from build123d import *

# Parameters (mm, degrees)
BOSS_EXTRUDE1_DEPTH  = 15
CUT_EXTRUDE1_START   = -4
SKETCH2_R            = 3
CUT_EXTRUDE1_DEPTH   = 17
M3_CLEARANCE_HOLE1_D = 3.4
FILLET2_R            = 2


with BuildPart() as part:
    # Sketch1 → Boss-Extrude1 (new body, symmetric)
    with BuildSketch(Plane(origin=(0, 0, 0), x_dir=(1, 0, 0), z_dir=(0, 1, 0))):
        Polygon((0, 0), (0, -7.5), (-20, 12.5), (-20, 25), (0, 5), align=None)
    extrude(amount=BOSS_EXTRUDE1_DEPTH, both=True)

    # Sketch2 → Cut-Extrude1 (cut, through all)
    with BuildSketch(Plane(origin=(0, 0, 0), x_dir=(0, 0, -1), z_dir=(1, 0, 0)).offset(CUT_EXTRUDE1_START)):
        with Locations((0, 10)):
            Circle(SKETCH2_R)
        with Locations((0, -10)):
            Circle(SKETCH2_R)
    extrude(amount=-CUT_EXTRUDE1_DEPTH, mode=Mode.SUBTRACT)

    # M3 Clearance Hole1 (through all)
    with Locations(Plane.ZY.offset(4)):
        with Locations((0, 10), (0, -10)):
            Hole(M3_CLEARANCE_HOLE1_D / 2)

    # Fillet2
    fillet2_edges = [part.edges().sort_by_distance(p)[0] for p in [
        (-20, 0, -12.5),
        (-20, 0, -25),
    ]]
    fillet(fillet2_edges, radius=FILLET2_R)


solid = part.part
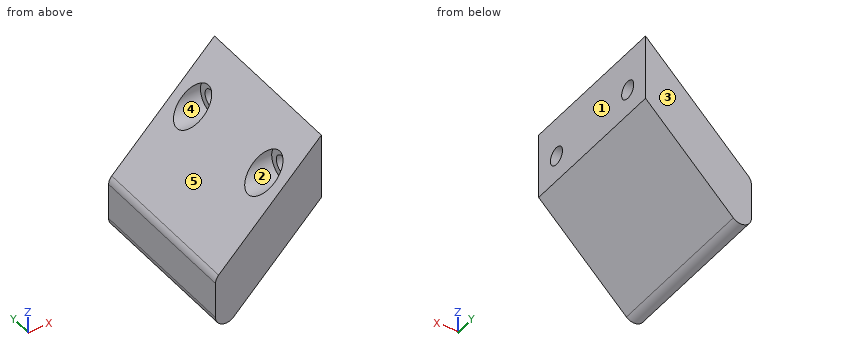
For this review, take the finished solid that the model builds, in its own axes (mm). Face numbers are marked on the shaded views. A direction names the side the tool comes from. Coordinates: 2 decimals unless noted, no trailing zeros. Order: outer loops, then holes, each group sorted by start corner. A loop starts at its lowest first (then second) coordinate and runs counter-clockwise, first axis right, second up. Notation, with made-up numbers: (-27.75, 39) -> (7.25, 39) arc R20 ccw to (7.25, 50) -> close; hole circle Ø5 at (-35, 11). An arc over 180 degrees is marked (long way). Return JSON: item names as keys, results as strings.
1. Machinability: for the marked faces 4 and 5, which of the approach directions +Z, -Z, +X, -X, +Y, -Y give a long, thin tool a straight path to every point of the face, cutting with its end or side? Answer none if there is none.
Answer block:
{"face 4": "-X", "face 5": "+Z, -X, +Y, -Y"}
2. We need section D-D on z = 4.5. Write out the cut boundary in (x, y).
Answer block:
{"outline": "(-3, -15) -> (0, -15) -> (0, 15) -> (-3, 15) -> close"}
3. We need section C-C on x = -4.75. Write out the cut boundary in (y, z), and give its area (3 significant figures).
Answer block:
{"outline": "(-15, -9.75) -> (15, -9.75) -> (15, 2.75) -> (11.2, 2.75) arc R3 cw (long way) to (8.8, 2.75) -> (-8.8, 2.75) arc R3 cw (long way) to (-11.2, 2.75) -> (-15, 2.75) -> close", "area": "319 mm²"}
4. The part is to be moulded in two halves that separate along Y. For the marked faces 1, 2 and 3, say which applies: +Y half, -Y half, draft (parallel to the pull), parting line (faces both ways), or undercut.
Answer block:
{"face 1": "draft", "face 2": "undercut", "face 3": "+Y half"}
5. We need section A-A on z = 0. Write out the cut boundary in (x, y).
Answer block:
{"outline": "(-7.5, -15) -> (0, -15) -> (0, -11.7) -> (-4, -11.7) -> (-4, -13) -> (-7.5, -13) -> close; (-7.5, -7) -> (-4, -7) -> (-4, -8.3) -> (0, -8.3) -> (0, 8.3) -> (-4, 8.3) -> (-4, 7) -> (-7.5, 7) -> close; (-7.5, 13) -> (-4, 13) -> (-4, 11.7) -> (0, 11.7) -> (0, 15) -> (-7.5, 15) -> close"}
6. We need section B-B on y = 10. Write out the cut boundary in (x, z), and give its area (3 significant figures).
Answer block:
{"outline": "(-20, -20.17) arc R2 ccw to (-16.59, -21.59) -> (0, -5) -> (0, -1.7) -> (-4, -1.7) -> (-4, -3) -> (-10.5, -3) -> (-19.41, -11.91) arc R2 ccw to (-20, -13.33) -> close; (-4.5, 3) -> (-4, 3) -> (-4, 1.7) -> (0, 1.7) -> (0, 7.5) -> close", "area": "210 mm²"}
7. For line 1 (Y direction, x = -1.85, z = 0); line 2 (X direction, y = -10.5, z = 2.75); line 3 (Z direction, x = -6, y = -1.5), list the stretches that pass through material, from the lowest coordinate up. Write a range as from..to.
Answer block:
{"line 1": "-15..-11.7, -8.3..8.3, 11.7..15", "line 2": "-4..0", "line 3": "-11..1.5"}
8. For pin 1 Ø8 at (y, z) = (10, 0) entering from +X; pin 2 Ø5.5 at (y, z) = (-10, 0) entering from -X; pin 3 Ø8 at (y, z) = (-1, 4.5) entering from -X; pin 4 Ø2 at (y, z) = (-3, -8.5) entering from -X, all flat-tipped, find the tip position at first contact; note any pin that passes through.
Answer block:
{"pin 1": "x = 0", "pin 2": "x = -4", "pin 3": "x = -7", "pin 4": "x = -17"}
